Geometry: final body of the model. Coordinates: model frame, mm. Face numbers are marked on the shaded views. Round coordinates to 2 decimals unless told otherwise and drop trailing zeros. Loops run counter-clockwise (first coordinate to the right, second up) from the corner with the lowest first, then second, coordinate; pieces in that order, holes last. Notation, with made-up numbers: M -26,36.25 L 2,36.25 A19 cw 2,48.25 Z; hole C 0.25,-13.75 d6. An arc over 180 degrees is marked long. Answer as a JSON object with one key per item and string values.
Autodesk Inventor part; units mm, degrees
ref_plane "YZ Plane" through (0, 0, 0) normal (1, 0, 0) x (0, 1, 0)
ref_plane "XZ Plane" through (0, 0, 0) normal (0, 1, 0) x (-1, 0, 0)
ref_plane "XY Plane" through (0, 0, 0) normal (0, 0, 1) x (1, 0, 0)
sketch "Sketch1" plane through (0, 0, 0) normal (0, 1, 0) x (-1, 0, 0)
  line L0 (100, -195) -> (-100, -195)
  line L1 (-100, -195) -> (-100, -255)
  line L2 (-100, -255) -> (100, -255)
  line L3 (100, -255) -> (100, -195)
  line L4 (0, 66.9735) -> (0, -172.2265)
  point P0 (0, 0)
  dimension "d0" = 200
  dimension "d1" = 60
  dimension "d2" = 195
extrude "Extrusion1" add sketch "Sketch1" along normal mid plane 650
chamfer "Chamfer1" distance 45 distance2 80 1 edges at (0, 325, -255) measured on face at (33.3333, 325, -215)
chamfer "Chamfer2" distance 45 distance2 80 1 edges at (0, -325, -255) measured on face at (33.3333, -325, -215)
sketch "Sketch2" plane through (0, -325, 0) normal (0, -1, 0) x (1, 0, 0)
  line L0 (100, -195) -> (-100, -195)
  line L1 (-80, -179) -> (-64, -179)
  line L2 (-64, -179) -> (-64, -195)
  line L3 (-64, -195) -> (-80, -195)
  line L4 (-80, -195) -> (-80, -179)
  line L5 (-100, -195) -> (-100, -210)
  line L6 (0, 0) -> (0, -427.5887)
  line L7 (80, -179) -> (64, -179)
  line L8 (64, -179) -> (64, -195)
  line L9 (64, -195) -> (80, -195)
  line L10 (80, -195) -> (80, -179)
  dimension "d11" = 20
  dimension "d12" = 16
  dimension "d13" = 16
extrude "Extrusion2" add sketch "Sketch2" against normal blind 650
sketch "Sketch3" plane through (100, -325, -195) normal (1, 0, 0) x (0, 0, -1)
  line L0 (-195, 325) -> (152.733, 325)
  line L1 (60, 80) -> (60, 570)
  line L2 (60, 193) -> (44, 193)
  line L3 (44, 193) -> (44, 213)
  line L4 (44, 213) -> (60, 213)
  line L5 (60, 213) -> (60, 193)
  line L6 (60, 457) -> (44, 457)
  line L7 (44, 457) -> (44, 437)
  line L8 (44, 437) -> (60, 437)
  line L9 (60, 437) -> (60, 457)
  point P0 (60, 437)
  point P1 (60, 213)
  dimension "d16" = 224
  dimension "d17" = 16
  dimension "d18" = 20
extrude "Extrusion3" cut sketch "Sketch3" against normal through all
properties part number "X_axis"
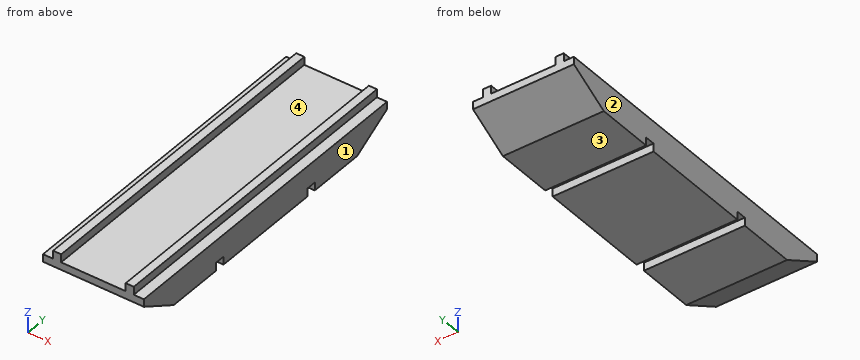
1) Cut plane C-C on y = 124. Return the cut outline in (x, z), and give its area (3 significant figures).
Geometry results:
{"outline": "M -100,-239 L 100,-239 L 100,-195 L 80,-195 L 80,-179 L 64,-179 L 64,-195 L -64,-195 L -64,-179 L -80,-179 L -80,-195 L -100,-195 Z", "area": "9,310 mm2"}
2) Cut plane D-D on z = -229.5. Return the cut outline in (x, y), and give its area (3 significant figures).
Geometry results:
{"outline": "M -100,-290.33 L 100,-290.33 L 100,290.33 L -100,290.33 Z", "area": "116,000 mm2"}
3) First-contact query: pin 1 (13 mm diameter, centred on x = 43, z = -245, fed in from +Y); pin 2 (8 mm diameter, centred on y = 141, z = -185.5, fed in from +X); pin 3 (6 mm diameter, centred on x = 92, y = 54, fed in from +Z). Flat tips, straight axial feed; report the tip coordinate or a pass-through.
Geometry results:
{"pin 1": "y = 274.33", "pin 2": "x = 80", "pin 3": "z = -195"}
4) Pull-direction query (X, two-part tool) for the marked faces 1, 2, 3 and 4; classes: +X half, -X half, draft (parallel to the pull), parting line (faces both ways), or undercut.
Geometry results:
{"face 1": "+X half", "face 2": "-X half", "face 3": "draft", "face 4": "undercut"}
5) Line query: probe 1 along Y at (x, z) = (-7.5, -249); probe 2 along Z at (x, y) = (34.5, -167.5); probe 3 along Z at (x, y) = (61.5, 115.5). Output: solid intervals per line, ascending.
Geometry results:
{"probe 1": "-255.67 to -132, -112 to 112, 132 to 255.67", "probe 2": "-255 to -195", "probe 3": "-239 to -195"}
6) Cut plane A-A on y = -97. Return the cut outline in (x, z), and give its area (3 significant figures).
Geometry results:
{"outline": "M -100,-255 L 100,-255 L 100,-195 L 80,-195 L 80,-179 L 64,-179 L 64,-195 L -64,-195 L -64,-179 L -80,-179 L -80,-195 L -100,-195 Z", "area": "12,500 mm2"}
7) Cut plane B-B on x = 4. Return the cut outline in (y, z).
Geometry results:
{"outline": "M -325,-210 L -245,-255 L -132,-255 L -132,-239 L -112,-239 L -112,-255 L 112,-255 L 112,-239 L 132,-239 L 132,-255 L 245,-255 L 325,-210 L 325,-195 L -325,-195 Z"}
